Design review of the part built by this model. Coordinates are the model's own, in mm. Face numbers are marked on the shaded views. A direction names the side the tool comes from. Coordinates: 2 decimals unless noted, no trailing zeros. Write each loop counter-clockwise with the first axis right and the second up, starting at its lowest first coordinate (ties: lowest second). Pieces come first, ordered by that corner, then holes. Notation, with made-up numbers: (77.5, -2.75) - (93.5, -2.75) arc R16 cw to (93.5, 24.25) - close; hole circle Ø4 at (-40, -19). An arc over 180 degrees is marked (long way). One line per item, written item: value.
Autodesk Inventor part; units mm, degrees
ref_plane "YZ Plane" through (0, 0, 0) normal (1, 0, 0) x (0, 1, 0)
ref_plane "XZ Plane" through (0, 0, 0) normal (0, 1, 0) x (-1, 0, 0)
ref_plane "XY Plane" through (0, 0, 0) normal (0, 0, 1) x (1, 0, 0)
sketch "Sketch1" plane through (0, 0, 0) normal (0, 0, 1) x (1, 0, 0)
  line L0 (0, 0) -> (0, -18)
  line L1 (0, -18) -> (-2, -18)
  line L2 (-2, -18) -> (-18, -2)
  line L3 (-18, -2) -> (-18, 0)
  line L4 (-18, 0) -> (0, 0)
  dimension "d0" = 18
  dimension "d1" = 2
extrude "Extrusion1" add sketch "Sketch1" along normal blind 2.5
sketch "Sketch2" plane through (0, 0, 2.5) normal (0, 0, 1) x (1, 0, 0)
  line L0 (0, -18) -> (0, 0)
  line L1 (0, 0) -> (-18, 0)
  line L2 (-18, 0) -> (-18, -2)
  line L3 (-18, -2) -> (-2, -18)
  line L4 (-2, -18) -> (0, -18)
  line L5 (-18, 0) -> (-18, -2)
  line L6 (-18, -2) -> (-2, -2)
  line L7 (-2, -18) -> (0, -18)
  line L8 (-2, -2) -> (-2, -18)
extrude "Extrusion2" add sketch "Sketch2" along normal blind 10 contours L4 L8 L6 L2 L1 L0
sketch "Sketch3" plane through (0, 0, 12.5) normal (0, 0, 1) x (1, 0, 0)
  line L0 (-2, -2) -> (-18, -2)
  line L1 (-18, -2) -> (-2, -18)
  line L2 (-2, -18) -> (-2, -2)
  line L3 (0, -18) -> (0, 0)
  line L4 (0, 0) -> (-18, 0)
  line L5 (-18, 0) -> (-18, -2)
  line L6 (-18, -2) -> (-2, -2)
  line L7 (-2, -2) -> (-2, -18)
  line L8 (-2, -18) -> (0, -18)
extrude "Extrusion3" add sketch "Sketch3" along normal blind 2.5
sketch "Sketch4" plane through (-18, 0, 0) normal (0, 1, 0) x (1, 0, 0)
  line L0 (0, 0) -> (18, 0)
  line L1 (0, 0) -> (0, -15)
  line L2 (18, -15) -> (0, -15)
  line L3 (18, 0) -> (18, -15)
  point P0 (7.5, -7.5)
  dimension "d8" = 7.5
  dimension "d9" = 7.5
hole "Hole1" at (-10.5, 0, 7.5) direction (0, -1, 0) diameter 3.7 depth 8 tip angle 118
sketch "Sketch5" plane through (0, -18, 0) normal (1, 0, 0) x (0, 0, -1)
  line L0 (0, 18) -> (0, 0)
  line L1 (0, 18) -> (-15, 18)
  line L2 (-15, 0) -> (-15, 18)
  line L3 (0, 0) -> (-15, 0)
  point P0 (-7.5, 7.5)
  dimension "d17" = 7.5
  dimension "d18" = 7.5
hole "Hole2" at (0, -10.5, 7.5) direction (-1, 0, 0) diameter 3.7 depth 8 tip angle 118
properties part number "Beam_CornerTri" material "ABS Plastic"
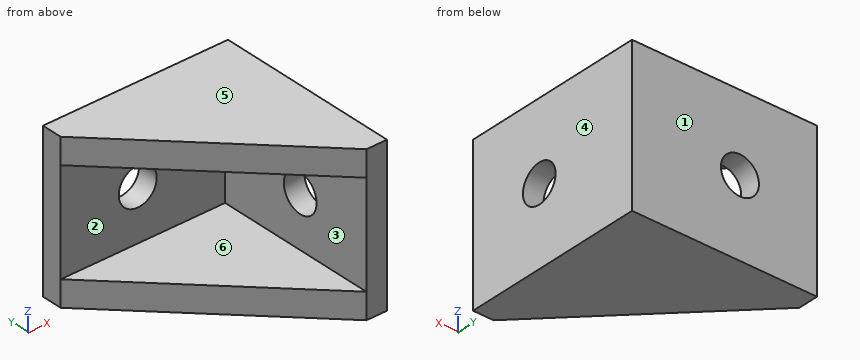
1. Insertion check: pin 1 Ø3 at (y, z) = (-3, 9.5) entering from -X; pin 2 Ø5 at (y, z) = (-9.5, 9) entering from -X; pin 3 Ø3 at (x, z) = (-8.5, 6.5) entering from -Y; pin 4 Ø4 at (y, z) = (-14, 3) entering from -X. Each pin has a flat end and moves straight along its axis. Give the tip position at first contact, or say it passes through.
Answer block:
pin 1: stops at x = -18
pin 2: stops at x = -2
pin 3: stops at y = -2
pin 4: stops at x = -7.94
2. Consider section B-B, the plane y = -10.5. Write out the cut boundary in (x, z).
Answer block:
outline: (-9.5, 0) - (0, 0) - (0, 5.65) - (-2, 5.65) - (-2, 2.5) - (-9.5, 2.5) - close; (-9.5, 12.5) - (-2, 12.5) - (-2, 9.35) - (0, 9.35) - (0, 15) - (-9.5, 15) - close
3. Consider section A-A, the plane z = 7.5. Write out the cut boundary in (x, y).
Answer block:
outline: (-18, -2) - (-12.35, -2) - (-12.35, 0) - (-18, 0) - close; (-8.65, -2) - (-2, -2) - (-2, -8.65) - (0, -8.65) - (0, 0) - (-8.65, 0) - close; (-2, -18) - (0, -18) - (0, -12.35) - (-2, -12.35) - close
4. Wall thickness on line 1 along Z through (x, y) = (-8.25, -6.25); line 2 along X through (y, z) = (-0.7, 7.5); line 3 along Z through (x, y) = (-0.65, -10.5): over which ranges is each line inside the solid? List them lowest first.
Answer block:
line 1: z = 0 to 2.5, 12.5 to 15
line 2: x = -18 to -12.35, -8.65 to 0
line 3: z = 0 to 5.65, 9.35 to 15
5. Consider section D-D, the plane y = -6.5. Write out the cut boundary in (x, z).
Answer block:
outline: (-13.5, 0) - (0, 0) - (0, 15) - (-13.5, 15) - (-13.5, 12.5) - (-2, 12.5) - (-2, 2.5) - (-13.5, 2.5) - close
6. Consider section C-C, the plane x = -14.75. Write out the cut boundary in (y, z), then the cut area to 4 significant figures.
Answer block:
outline: (-5.25, 0) - (0, 0) - (0, 15) - (-5.25, 15) - (-5.25, 12.5) - (-2, 12.5) - (-2, 2.5) - (-5.25, 2.5) - close
area: 46.25 mm^2
7. For the marked faces 1 and 2, list the 3-axis set-ups (+Z, -Z, +X, -X, +Y, -Y) from which the entire face can be reached by the end or side of a thin tool; tool diameter is ignored.
Answer block:
face 1: +Z, -Z, +X, -X, +Y
face 2: -X, -Y
8. Mouldability with a two-part tool opening along Z and no side actions: class the marked faces 3, 4, 5 and 6 as released by +Z, released by -Z, zero draft, split by the parting line, or undercut.
Answer block:
face 3: undercut
face 4: zero draft
face 5: released by +Z
face 6: undercut
